Input: part model. Units: mm. Frame: model coordinates. Coordinates: 2 decimals unless noted, no trailing zeros.
```python
from build123d import *

# Parameters (mm, degrees)
BOSS_EXTRUDE1_DEPTH = 76.2
CIRPATTERN1_COUNT   = 4


with BuildPart() as part:
    # Sketch3 → Boss-Extrude1 (new body, symmetric)
    with BuildSketch(Plane.XY):
        with BuildLine():
            Line((-4.503841895, 3.156803476), (-3.14772708, 1.530298739))
            ThreePointArc((-3.14772708, 1.530298739), (-3.410794979, 0.785160882), (-3.5, 0))
            Line((-3.5, 0), (-5.5, 0))
            Line((-5.5, 0), (-6, 0.866025404))
            Line((-6, 0.866025404), (-6, 3.996841995))
            ThreePointArc((-6, 3.996841995), (-6.038060234, 4.188183711), (-6.146446609, 4.350395385))
            Line((-6.146446609, 4.350395385), (-9.917104615, 8.121053391))
            ThreePointArc((-9.917104615, 8.121053391), (-10.079316289, 8.229439766), (-10.270658005, 8.2675))
            Line((-10.270658005, 8.2675), (-12.29, 8.2675))
            ThreePointArc((-12.29, 8.2675), (-12.643553391, 8.121053391), (-12.79, 7.7675))
            Line((-12.79, 7.7675), (-12.79, 4.5))
            ThreePointArc((-12.79, 4.5), (-12.936446609, 4.146446609), (-13.29, 4))
            Line((-13.29, 4), (-14.5, 4))
            Line((-14.5, 4), (-14.5, 4.5))
            Line((-14.5, 4.5), (-15, 4.5))
            Line((-15, 4.5), (-15, 12.968))
            ThreePointArc((-15, 12.968), (-14.404840979, 14.404840979), (-12.968, 15))
            Line((-12.968, 15), (-4.5, 15))
            Line((-4.5, 15), (-4.5, 14.5))
            Line((-4.5, 14.5), (-4, 14.5))
            Line((-4, 14.5), (-4, 13.29))
            ThreePointArc((-4, 13.29), (-4.146446609, 12.936446609), (-4.5, 12.79))
            Line((-4.5, 12.79), (-7.7675, 12.79))
            ThreePointArc((-7.7675, 12.79), (-8.121053391, 12.643553391), (-8.2675, 12.29))
            Line((-8.2675, 12.29), (-8.2675, 10.270658005))
            ThreePointArc((-8.2675, 10.270658005), (-8.229439766, 10.079316289), (-8.121053391, 9.917104615))
            Line((-8.121053391, 9.917104615), (-4.350395385, 6.146446609))
            ThreePointArc((-4.350395385, 6.146446609), (-4.188183711, 6.038060234), (-3.996841995, 6))
            Line((-3.996841995, 6), (-0.866025404, 6))
            Line((-0.866025404, 6), (0, 5.5))
            Line((0, 5.5), (0, 3.5))
            ThreePointArc((0, 3.5), (-0.785160882, 3.410794979), (-1.530298739, 3.14772708))
            Line((-1.530298739, 3.14772708), (-3.156803476, 4.503841895))
            ThreePointArc((-3.156803476, 4.503841895), (-3.889087297, 3.889087297), (-4.503841895, 3.156803476))
        make_face()
        with BuildLine():
            Line((-12.705, 9.5135), (-10.5135, 9.5135))
            ThreePointArc((-10.5135, 9.5135), (-9.806393219, 9.806393219), (-9.5135, 10.5135))
            Line((-9.5135, 10.5135), (-9.5135, 12.705))
            ThreePointArc((-9.5135, 12.705), (-9.806393219, 13.412106781), (-10.5135, 13.705))
            Line((-10.5135, 13.705), (-12.705, 13.705))
            ThreePointArc((-12.705, 13.705), (-13.412106781, 13.412106781), (-13.705, 12.705))
            Line((-13.705, 12.705), (-13.705, 10.5135))
            ThreePointArc((-13.705, 10.5135), (-13.412106781, 9.806393219), (-12.705, 9.5135))
        make_face(mode=Mode.SUBTRACT)
    boss_extrude1 = extrude(amount=BOSS_EXTRUDE1_DEPTH, both=True)

    # CirPattern1: Boss-Extrude1 ×4 about axis
    cirpattern1_axis = Axis((0, 0, 0), (0, 0, 1))
    for i in range(1, CIRPATTERN1_COUNT):
        add(boss_extrude1.rotate(cirpattern1_axis, i * 360 / CIRPATTERN1_COUNT))


solid = part.part
```
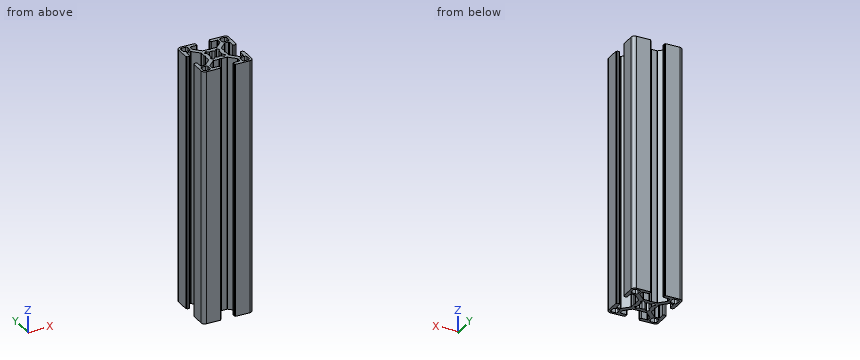
Item 1: Section query A-A (z = -63.5). Count the separate pieces of the cut face and the enclosed holes in it, then the cut area to 3 significant figures.
Result:
separate pieces: 1
enclosed holes: 5
area: 317 mm2
Item 2: Contact query for flat-ended pins moving along their axis: P1, Ø1.3, axis at x = -14, z = 26.5, coming from the +Y side; P2, Ø0.6, axis at x = 15, z = 22.5, coming from the +Y side; P3, Ø1.5, axis at x = -1, z = -27.5, coming from the +Y side. Output: stop coordinate, or through.
Result:
P1: stops at y = 14.96
P2: stops at y = 14.03
P3: stops at y = 6
Item 3: Line query: L1, parallel to X at y = -10.75, z = -41.5 (1 decimal); L2, parallel to Y at x = -3, z = 27.5; L3, parallel to X at y = 10, z = -13.5. Output: solid intervals per line, ascending.
Result:
L1: x = -15 to -13.7, -9.5 to -8.3, 8.3 to 9.5, 13.7 to 15
L2: y = -6 to -4.37, 4.37 to 6
L3: x = -15 to -13.56, -9.66 to -8.19, 8.19 to 9.66, 13.56 to 15
